Here's how the part is built. I have some questions about the finished solid (model axes, mm). A direction names the side the tool comes from. Coordinates: 2 decimals unless noted, no trailing zeros. Loops run counter-clockwise (first coordinate to the right, second up) from the corner with the lowest first, then second, coordinate; pieces in that order, holes last. Notation, with made-up numbers: M 69,19 L 114,19 A16 cw 114,26 Z; hole C -32,8 d4. An arc over 180 degrees is marked long. Use one line per item in the form item = value. Start each with the question number.
(1) Will these pins go through, and if not, where does the flat tip stop? P1, Ø1, axis at y = 1, z = -3, coming from the +X side; P2, Ø1.8, axis at x = 10, y = 1.5, coming from the -Z side; P3, Ø1, axis at x = 0, y = -2, coming from the +Z side.
(2) Please list where these lines run through material, in increasing order: L1, parallel to Z at x = -7.75, y = -0.1; L2, parallel to X at y = -2.1, z = -2.5; L3, parallel to Z at x = -10.5, y = -2.1.
(3) On a 3-axis mill with a long thin cutter (end or side, diameter ignored), from which of +Z, -Z, +X, -X, +Y, -Y can I reach the whole of each face in a straight line? I mean faces 5 (the flat face through (-9, 0, -1.588)), 6 (the cylindrical face through (-10.355, -0.042, -0.238)), 7 (the flat face through (9, 0, -1.588)). Say none if no direction works.
(4) Imagine slicing it at C-C, the plane x = -9.25. Please give me the cut outline in (y, z).
(5) Imagine slicing it at B-B, the plane x = 0. Please give me the cut outline in (y, z) (1 decimal), and give its area (4 significant figures).
(6) Imagine slicing it at A-A, the plane y = -1.7. State how many separate pieces and enclosed holes the cut face has, and give its area (3 significant figures).
(7) Thinking about a two-plate mould opening in X: for faces 1 (the flat face through (-14.288, 0, 0)), 2 (the cylindrical face through (-0.07, 0.042, -3.174)), 3 (the flat face through (14.288, 0, 0)), 4 (the flat face through (10, 0, 1.588)), which applies, +X half, -X half, draft (parallel to the pull), parting line (faces both ways), or undercut?
```python
from build123d import *

# Parameters (mm, degrees)
SKETCH1_R           = 0.79375
BOSS_EXTRUDE1_DEPTH = 3


with BuildPart() as part:
    # Sketch1 → Boss-Extrude1 (new body, symmetric)
    with BuildSketch(Plane(origin=(0, 0, 0), x_dir=(1, 0, 0), z_dir=(0, 1, 0))):
        with BuildLine():
            ThreePointArc((-4.682314967, -0.870248702), (-4.742411374, -0.436967517), (-4.7625, 0))
            ThreePointArc((-4.7625, 0), (-4.69391314, 0.805348174), (-4.490128061, 1.5875))
            Line((-4.490128061, 1.5875), (-14.2875, 1.5875))
            Line((-14.2875, 1.5875), (-14.2875, -1.5875))
            Line((-14.2875, -1.5875), (-5.924630657, -1.5875))
            Line((-5.924630657, -1.5875), (-4.682314967, -0.870248702))
        make_face()
        with Locations((-11.1125, 0)):
            Circle(SKETCH1_R, mode=Mode.SUBTRACT)
        with BuildLine():
            Line((-4.7625, 0), (-3.175, 0))
            ThreePointArc((-3.175, 0), (-3.066814498, 0.821750468), (-2.749630657, 1.5875))
            Line((-2.749630657, 1.5875), (-4.490128061, 1.5875))
            ThreePointArc((-4.490128061, 1.5875), (-4.69391314, 0.805348174), (-4.7625, 0))
        make_face()
        with BuildLine():
            ThreePointArc((-2.749630657, 1.5875), (0, 3.175), (2.749630657, 1.5875))
            Line((2.749630657, 1.5875), (4.490128061, 1.5875))
            ThreePointArc((4.490128061, 1.5875), (0, 4.7625), (-4.490128061, 1.5875))
            Line((-4.490128061, 1.5875), (-2.749630657, 1.5875))
        make_face()
        with BuildLine():
            ThreePointArc((2.749630657, 1.5875), (3.066814498, 0.821750468), (3.175, 0))
            Line((3.175, 0), (4.7625, 0))
            ThreePointArc((4.7625, 0), (4.69391314, 0.805348174), (4.490128061, 1.5875))
            Line((4.490128061, 1.5875), (2.749630657, 1.5875))
        make_face()
        with BuildLine():
            ThreePointArc((4.490128061, 1.5875), (4.69391314, 0.805348174), (4.7625, 0))
            ThreePointArc((4.7625, 0), (4.742411374, -0.436967517), (4.682314967, -0.870248702))
            Line((4.682314967, -0.870248702), (5.924630657, -1.5875))
            Line((5.924630657, -1.5875), (14.2875, -1.5875))
            Line((14.2875, -1.5875), (14.2875, 1.5875))
            Line((14.2875, 1.5875), (4.490128061, 1.5875))
        make_face()
        with Locations((11.1125, 0)):
            Circle(SKETCH1_R, mode=Mode.SUBTRACT)
        with BuildLine():
            Line((-4.682314967, -0.870248702), (-3.175, 0))
            Line((-3.175, 0), (-4.7625, 0))
            ThreePointArc((-4.7625, 0), (-4.742411374, -0.436967517), (-4.682314967, -0.870248702))
        make_face()
        with BuildLine():
            Line((4.7625, 0), (3.175, 0))
            Line((3.175, 0), (4.682314967, -0.870248702))
            ThreePointArc((4.682314967, -0.870248702), (4.742411374, -0.436967517), (4.7625, 0))
        make_face()
    extrude(amount=BOSS_EXTRUDE1_DEPTH, both=True)


solid = part.part
```
Answer:
q1.P1 = 4.05
q1.P2 = -1.59
q1.P3 = -3.14
q2.L1 = -1.59 to 1.59
q2.L2 = -4.05 to -1.96, 1.96 to 4.05
q2.L3 = -1.59 to -0.5, 0.5 to 1.59
q3.face_5 = -Z, -X, +Y, -Y
q3.face_6 = +Y, -Y
q3.face_7 = -Z, +X, +Y, -Y
q4.outline = M -3,-1.59 L 3,-1.59 L 3,1.59 L -3,1.59 Z
q5.outline = M -3,-4.8 L 3,-4.8 L 3,-3.2 L -3,-3.2 Z
q5.area = 9.525 mm²
q6.separate_pieces = 1
q6.enclosed_holes = 2
q6.area = 77.3 mm²
q7.face_1 = -X half
q7.face_2 = undercut
q7.face_3 = +X half
q7.face_4 = draft
